Part model, mm, in its own coordinate system. Face numbers are marked on the shaded views. A direction names the side the tool comes from. Give positions to 0.01 mm unless a question says otherwise; leave off trailing zeros. Write each loop counter-clockwise with the first axis right and the second up, starting at its lowest first coordinate (ties: lowest second). Pieces come first, ordered by that corner, then holes.
Autodesk Inventor part; units mm, degrees
ref_plane "YZ Plane" through (0, 0, 0) normal (1, 0, 0) x (0, 1, 0)
ref_plane "XZ Plane" through (0, 0, 0) normal (0, 1, 0) x (-1, 0, 0)
ref_plane "XY Plane" through (0, 0, 0) normal (0, 0, 1) x (1, 0, 0)
sketch "Sketch1" plane through (0, 0, 0) normal (0, 1, 0) x (-1, 0, 0)
  line L0 (50.3036, 45.5466) -> (-49.6964, 45.5466)
  line L1 (-49.6964, 45.5466) -> (-49.6964, -54.4534)
  line L2 (-49.6964, -54.4534) -> (50.3036, -54.4534)
  line L3 (50.3036, -54.4534) -> (50.3036, 45.5466)
  point P0 (0, 0)
  dimension "d0" = 100
  dimension "d1" = 100
extrude "Extrusion1" add sketch "Sketch1" along normal blind 50
fillet "Fillet1" radius 3 8 edges at (49.6964, 50, -4.4534) (-0.3036, 50, 45.5466) (49.6964, 25, 45.5466) (-50.3036, 25, 45.5466) (-50.3036, 50, -4.4534) (-0.3036, 50, -54.4534) (49.6964, 25, -54.4534) (-50.3036, 25, -54.4534)
shell "Shell1" thickness 3 removed faces 1 at (14.363, 0, 11.2132)
sketch "Sketch2" plane through (0, 50, 0) normal (0, 1, 0) x (1, 0, 0)
  circle A0 centre (-0.3036, 4.4534) radius 28
  line L0 (-47.3036, -45.5466) -> (46.6964, -45.5466)
  line L1 (-50.3036, 51.4534) -> (-50.3036, -42.5466)
  point P0 (0, 0)
  dimension "d6" = 56
  dimension "d7" = 50
  dimension "d8" = 50
extrude "Extrusion2" cut sketch "Sketch2" against normal blind 50
properties part number "Top"
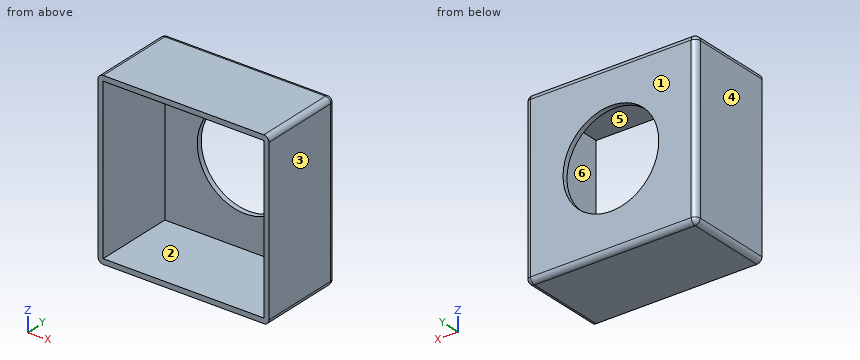
1) Flat gauge pin, fed straight in: P1, Ø6, axis at x = 21.5, z = -22, coming from the -Y side. Where does the tip first touch, or does it go through?
Check result:
P1: stops at y = 47
2) Mould opens along X. For the marked faces 3, 4, 5 and 6 say: +X half, -X half, draft (parallel to the pull), parting line (faces both ways), or undercut.
Check result:
face 3: +X half
face 4: -X half
face 5: undercut
face 6: undercut
3) Saw through at D-D (z = 0). Write the cut outline in (x, y).
Check result:
outline: (-50.3, 0) - (-47.3, 0) - (-47.3, 47) - (-27.95, 47) - (-27.95, 50) - (-47.3, 50) arc R3 ccw to (-50.3, 47) - close; (27.34, 47) - (46.7, 47) - (46.7, 0) - (49.7, 0) - (49.7, 47) arc R3 ccw to (46.7, 50) - (27.34, 50) - close
4) Saw through at B-B (x = 25.5). Write the cut outline in (y, z).
Check result:
outline: (0, -54.45) - (47, -54.45) arc R3 ccw to (50, -51.45) - (50, -15.32) - (47, -15.32) - (47, -51.45) - (0, -51.45) - close; (0, 42.55) - (47, 42.55) - (47, 6.42) - (50, 6.42) - (50, 42.55) arc R3 ccw to (47, 45.55) - (0, 45.55) - close
5) Drill centre lines: L1, parallel to Z at x = -7, y = 45.5; L2, parallel to X at y = 11, z = 0; L3, parallel to Y at x = 32, z = -17. Where is each one in solid material? Low to high.
Check result:
L1: z = -54.45 to -51.45, 42.55 to 45.55
L2: x = -50.3 to -47.3, 46.7 to 49.7
L3: y = 47 to 50
6) 3-axis set-ups, long thin cutter, end or side, ignore diameter. For the marked faces 1 and 2: which of +Z, -Z, +X, -X, +Y, -Y reach the whole face in a straight line?
Check result:
face 1: +Z, -Z, +X, -X, +Y
face 2: -Y
7) Saw through at C-C (z = 28). Write the cut outline in (x, y), and give its area (3 significant figures).
Check result:
outline: (-50.3, 0) - (-47.3, 0) - (-47.3, 47) - (46.7, 47) - (46.7, 0) - (49.7, 0) - (49.7, 47) arc R3 ccw to (46.7, 50) - (-47.3, 50) arc R3 ccw to (-50.3, 47) - close
area: 578 mm2
8) Saw through at A-A (y = 14). Write the cut outline in (x, z), and give its area (3 significant figures).
Check result:
outline: (-50.3, -51.45) arc R3 ccw to (-47.3, -54.45) - (46.7, -54.45) arc R3 ccw to (49.7, -51.45) - (49.7, 42.55) arc R3 ccw to (46.7, 45.55) - (-47.3, 45.55) arc R3 ccw to (-50.3, 42.55) - close; hole (-47.3, -51.45) - (46.7, -51.45) - (46.7, 42.55) - (-47.3, 42.55) - close
area: 1,160 mm2
